Can you work these out from the drawing? Everything is in mm from the part's minimum corner. Coordinates: 2 decimals unless noted, no trailing zeros. Order: outer loops, then holes, each group sorted by start corner. A loop starts at its lowest first (then second) coordinate and runs counter-clockwise, first axis right, second up. Notation, with made-up numbers: M -1.5,73 L 32.5,73 A31 ccw 32.5,100 Z; hole C 35,24.5 d4. An arc over 180 degrees is marked long. Answer as a JSON object with one key per item and string values.
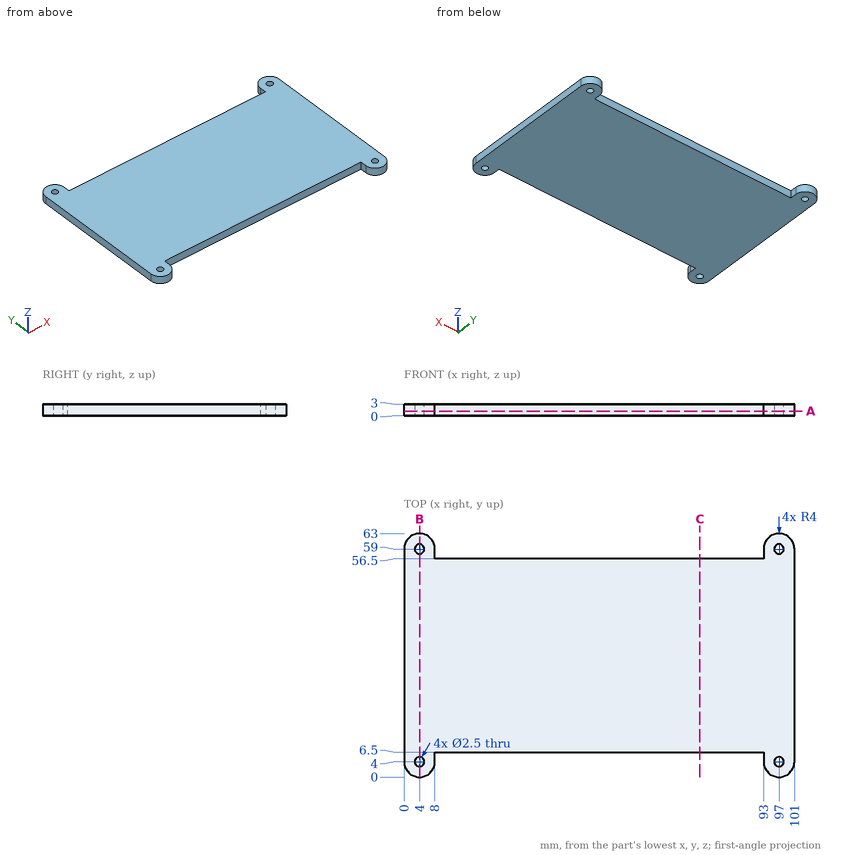
Item 1: I want a section at C-C, the plane x = 76.5. Write out the boundary of the cut face in (y, z), plus the area to 3 significant figures.
Answers follow:
{"outline": "M 6.5,0 L 56.5,0 L 56.5,3 L 6.5,3 Z", "area": "150 mm^2"}
Item 2: I want a section at B-B, the plane x = 4. Write out the boundary of the cut face in (y, z).
Answers follow:
{"outline": "M 0,0 L 2.75,0 L 2.75,3 L 0,3 Z; M 5.25,0 L 57.75,0 L 57.75,3 L 5.25,3 Z; M 60.25,0 L 63,0 L 63,3 L 60.25,3 Z"}
Item 3: Please list where these lines run through material, in increasing order: line 1 (Y direction, x = 97, z = 1.3); line 2 (X direction, y = 59, z = 0.75); line 3 (Y direction, x = 96.5, z = 1.4).
Answers follow:
{"line 1": "y = 0 to 2.75, 5.25 to 57.75, 60.25 to 63", "line 2": "x = 0 to 2.75, 5.25 to 8, 93 to 95.75, 98.25 to 101", "line 3": "y = 0.03 to 2.85, 5.15 to 57.85, 60.15 to 62.97"}
Item 4: I'm going to push a flat-ended pin straight in: pin 1 (0.9 mm diameter, centred on x = 60, z = 1, fed in from +Y). Where does the tip first touch, or does it pass through?
Answers follow:
{"pin 1": "stops at y = 56.5"}
Item 5: I want a section at A-A, the plane z = 1.15. Write out the boundary of the cut face in (x, y), plus the area to 3 significant figures.
Answers follow:
{"outline": "M 0,4 A4 ccw 8,4 L 8,6.5 L 93,6.5 L 93,4 A4 ccw 101,4 L 101,59 A4 ccw 93,59 L 93,56.5 L 8,56.5 L 8,59 A4 ccw 0,59 Z; hole C 4,4 d2.5; hole C 4,59 d2.5; hole C 97,4 d2.5; hole C 97,59 d2.5", "area": "5,210 mm^2"}
